```python
from build123d import *

# Parameters (mm, degrees)
F0_R          = 10.5
F1_DEPTH      = 18.5
F3_DEPTH      = 16.5
F4_R          = 9.75
F5_DEPTH      = 6
F6_R          = 2.5
F7_DEPTH      = 10.501
F7_DEPTH_BACK = 10.501


with BuildPart() as f1:
    # F0 (on Top) → F1 (new body)
    with BuildSketch(Plane.XY):
        Circle(F0_R)
    extrude(amount=F1_DEPTH)

    # F2 (on face) → F3 (cut)
    with BuildSketch(Plane(origin=(0, 0, 0), x_dir=(1, 0, 0), z_dir=(0, 0, -1))):
        with BuildLine():
            Line((2.75, 6.25), (-2.75, 6.25))
            ThreePointArc((-2.75, 6.25), (-9, 0), (-2.75, -6.25))
            Line((-2.75, -6.25), (2.75, -6.25))
            ThreePointArc((2.75, -6.25), (9, 0), (2.75, 6.25))
        make_face()
    extrude(amount=-F3_DEPTH, mode=Mode.SUBTRACT)

    # F4 (on face) → F5 (cut)
    with BuildSketch(Plane(origin=(0, 0, 0), x_dir=(1, 0, 0), z_dir=(0, 0, -1))):
        Circle(F4_R)
        with BuildLine():
            Line((-2.75, 6.25), (2.75, 6.25))
            ThreePointArc((2.75, 6.25), (9, 0), (2.75, -6.25))
            Line((2.75, -6.25), (-2.75, -6.25))
            ThreePointArc((-2.75, -6.25), (-9, 0), (-2.75, 6.25))
        make_face(mode=Mode.SUBTRACT)
    extrude(amount=-F5_DEPTH, mode=Mode.SUBTRACT)

    # F6 (on Front) → F7 (cut, two sides)
    with BuildSketch(Plane.XZ) as f7_sk:
        with Locations((0, 10.5)):
            Circle(F6_R)
    extrude(amount=-F7_DEPTH, mode=Mode.SUBTRACT)
    extrude(f7_sk.sketch, amount=F7_DEPTH_BACK, mode=Mode.SUBTRACT)


solid = f1.part
```
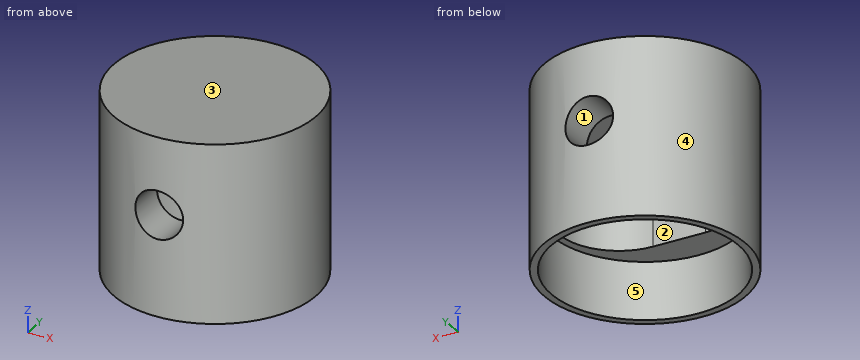
Check sheet for the modelled part. Datum: model origin and axes. Units: mm. Face numbers are marked on the shaded views. A direction names the side the tool comes from. Round coordinates to 2 decimals unless told otherwise and drop trailing zeros. Loops run counter-clockwise (first coordinate to the right, second up) from the corner with the lowest first, then second, coordinate; pieces in that order, holes last. Notation, with made-up numbers: M -12.5,-7 L -2.5,-7 A4 cw -2.5,-1 Z; hole C -19,-34.75 d1. An arc over 180 degrees is marked long. Answer as a JSON object with one key per item and string values.
1. Access from +Z, -Z, +X, -X, +Y, -Y to the whole of each face (thin tool, end or side, straight path). Record for the marked faces 1 and 2.
Reply:
{"face 1": "+Y, -Y", "face 2": "-Z"}
2. Gauge pin test, flat ends, axial feed: P1, Ø1, axis at x = 3.5, z = 7, coming from the +Y side; P2, Ø6.5, axis at x = 3.5, y = 0, coming from the -Z side; P3, Ø1, axis at x = 7.5, z = 7.5, coming from the -Y side. Record the tip position at first contact, or that the pin passes through.
Reply:
{"P1": "stops at y = 10.06", "P2": "stops at z = 16.5", "P3": "stops at y = -7.83"}
3. Mould release check, pull along Y, two halves, no side actions. Record for the marked faces 3, 4 and 5: pulls with the +Y half, pulls with the -Y half, needs draft (parallel to the pull), parting line crosses it, or undercut.
Reply:
{"face 3": "needs draft", "face 4": "parting line crosses it", "face 5": "undercut"}
4. Section check A-A (z = 12.25). Record the boundary of the cut face in (x, y), plus the area to 3 significant figures.
Reply:
{"outline": "M -2.75,-6.25 A6.25 cw -2.75,6.25 L -1.79,6.25 L -1.79,10.35 A10.5 ccw -1.79,-10.35 L -1.79,-6.25 Z; M 1.79,-10.35 A10.5 ccw 1.79,10.35 L 1.79,6.25 L 2.75,6.25 A6.25 cw 2.75,-6.25 L 1.79,-6.25 Z", "area": "125 mm²"}
5. Section check B-B (x = 0). Record the boundary of the cut face in (y, z).
Reply:
{"outline": "M -10.5,0 L -9.75,0 L -9.75,6 L -6.25,6 L -6.25,8 L -10.5,8 Z; M -10.5,13 L -6.25,13 L -6.25,16.5 L 6.25,16.5 L 6.25,13 L 10.5,13 L 10.5,18.5 L -10.5,18.5 Z; M 6.25,6 L 9.75,6 L 9.75,0 L 10.5,0 L 10.5,8 L 6.25,8 Z"}
6. Section check D-D (z = 14.75). Record the boundary of the cut face in (x, y).
Reply:
{"outline": "C 0,0 d21; hole M -2.75,-6.25 L 2.75,-6.25 A6.25 ccw 2.75,6.25 L -2.75,6.25 A6.25 ccw Z"}
7. Section check C-C (y = 0). Record the boundary of the cut face in (x, z).
Reply:
{"outline": "M -10.5,0 L -9.75,0 L -9.75,6 L -9,6 L -9,16.5 L 9,16.5 L 9,6 L 9.75,6 L 9.75,0 L 10.5,0 L 10.5,18.5 L -10.5,18.5 Z"}
8. Scan lines: line 1 (Z direction, x = 0, y = 9.45); line 2 (Y direction, x = 0, z = 1.6); line 3 (Z direction, x = 1.5, y = -5). Record each from-to range of solid material in increasing order.
Reply:
{"line 1": "z = 6 to 8, 13 to 18.5", "line 2": "y = -10.5 to -9.75, 9.75 to 10.5", "line 3": "z = 16.5 to 18.5"}
